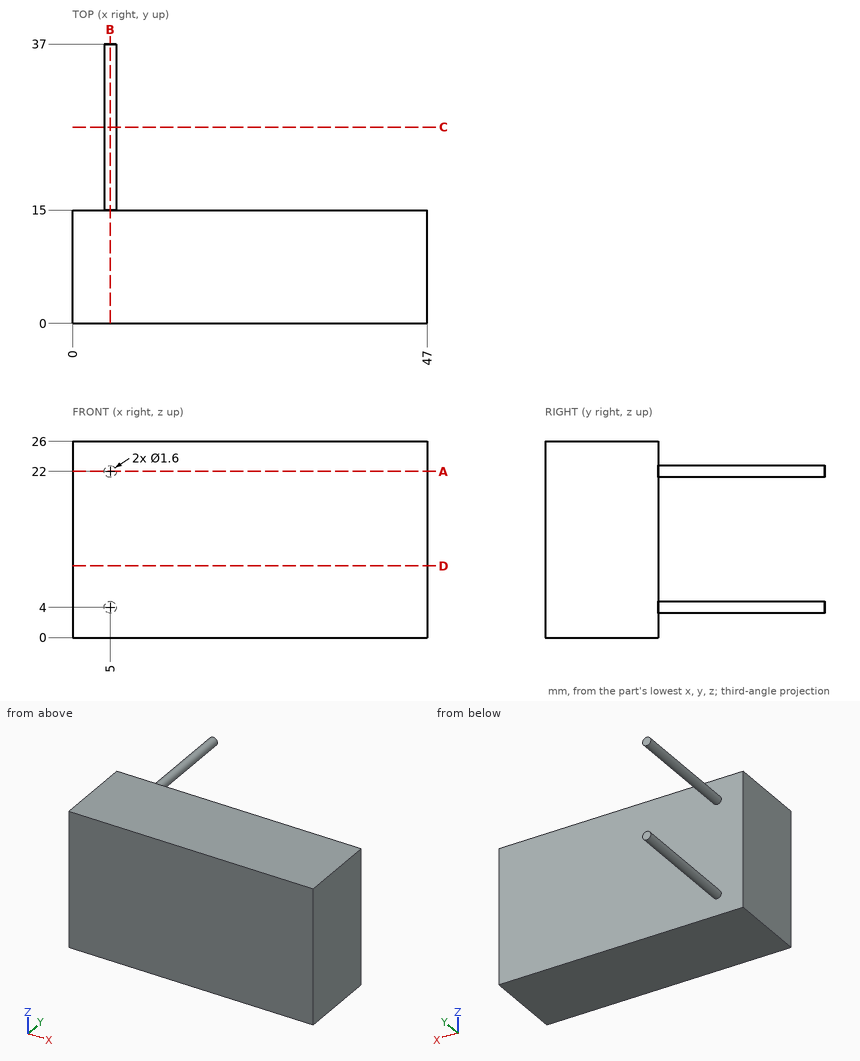
Print and shaded views of the part. All mm, measured from the part's lowest x, y and z. Round coordinates to 2 decimals unless told otherwise and drop trailing zeros. Order: outer loops, then holes, each group sorted by start corner. A loop starts at its lowest first (then second) coordinate and runs counter-clockwise, first axis right, second up.
Q1. Slice it at B-B (x = 5). Write the cut outline in (y, z).
Q2. Slice it at C-C (y = 26). Write the cut outline in (x, z).
Q3. Slice it at A-A (z = 22). Write the cut outline in (x, y), and give its area (3 significant figures).
Q4. Drop flat-ended pins along their axis: pin 1 (6 mm diameter, centred on x = 5, z = 7, fed in from +Y); pin 2 (8 mm diameter, centred on x = 21.5, z = 16.5, fed in from +Y); pin 3 (2 mm diameter, centred on y = 17.5, z = 22.5, fed in from +X). Give the stop position or say it passes through.
Q5. Slice it at D-D (z = 9.5). Write the cut outline in (x, y).
Q6. Wall check: L1, parallel to Y at x = 41, z = 13; L2, parallel to X at y = 30.5, z = 4.25. Give the ranges that are in metal, low to high.
Results below:
1. outline: (0, 0) - (15, 0) - (15, 3.2) - (37, 3.2) - (37, 4.8) - (15, 4.8) - (15, 21.2) - (37, 21.2) - (37, 22.8) - (15, 22.8) - (15, 26) - (0, 26) - close
2. outline: circle Ø1.6 at (5, 4); circle Ø1.6 at (5, 22)
3. outline: (0, 0) - (47, 0) - (47, 15) - (5.8, 15) - (5.8, 37) - (4.2, 37) - (4.2, 15) - (0, 15) - close
3. area: 740 mm2
4. pin 1: stops at y = 37
4. pin 2: stops at y = 15
4. pin 3: stops at x = 5.8
5. outline: (0, 0) - (47, 0) - (47, 15) - (0, 15) - close
6. L1: y = 0 to 15
6. L2: x = 4.24 to 5.76
